```python
from build123d import *

# Parameters (mm, degrees)
BOSS_EXTRUDE1_DEPTH = 6
SKETCH2_R           = 1.125
SKETCH2_R_2         = 1.35
CUT_EXTRUDE1_DEPTH  = 7


with BuildPart() as part:
    # Sketch1 → Boss-Extrude1 (new body)
    with BuildSketch(Plane(origin=(0, 0, 0), x_dir=(1, 0, 0), z_dir=(0, 1, 0))):
        with BuildLine():
            Line((-12, 3.875), (12, 3.875))
            ThreePointArc((12, 3.875), (14.121320344, 2.996320344), (15, 0.875))
            Line((15, 0.875), (15, -0.875))
            ThreePointArc((15, -0.875), (14.121320344, -2.996320344), (12, -3.875))
            Line((12, -3.875), (-12, -3.875))
            ThreePointArc((-12, -3.875), (-14.121320344, -2.996320344), (-15, -0.875))
            Line((-15, -0.875), (-15, 0.875))
            ThreePointArc((-15, 0.875), (-14.121320344, 2.996320344), (-12, 3.875))
        make_face()
    extrude(amount=BOSS_EXTRUDE1_DEPTH)

    # Sketch2 → Cut-Extrude1 (cut, through all)
    with BuildSketch(Plane(origin=(0, 6, 0), x_dir=(1, 0, 0), z_dir=(0, 1, 0))):
        with Locations((-10, 0)):
            Circle(SKETCH2_R)
        with Locations((10, 0)):
            Circle(SKETCH2_R_2)
    extrude(amount=-CUT_EXTRUDE1_DEPTH, mode=Mode.SUBTRACT)


solid = part.part
```
The model under review builds one solid part; all positions refer to its coordinate system, in mm. Round coordinates to 2 decimals unless told otherwise and drop trailing zeros. Loops run counter-clockwise (first coordinate to the right, second up) from the corner with the lowest first, then second, coordinate; pieces in that order, holes last.
1) Consider section C-C on y = 1.1. State the section outline as (x, z) points (3 decimals), then the cut area to 3 significant figures.
Values follow:
outline: (-15, -0.875) arc R3 ccw to (-12, -3.875) - (12, -3.875) arc R3 ccw to (15, -0.875) - (15, 0.875) arc R3 ccw to (12, 3.875) - (-12, 3.875) arc R3 ccw to (-15, 0.875) - close; hole circle Ø2.25 at (-10, 0); hole circle Ø2.7 at (10, 0)
area: 215 mm2
2) Consider section B-B on z = 0. State the section outline as (x, y) points (3 decimals), then the cut area to 3 significant figures.
Values follow:
outline: (-15, 0) - (-11.125, 0) - (-11.125, 6) - (-15, 6) - close; (-8.875, 0) - (8.65, 0) - (8.65, 6) - (-8.875, 6) - close; (11.35, 0) - (15, 0) - (15, 6) - (11.35, 6) - close
area: 150 mm2
3) The part is to be moulded in two halves that separate along Z. For faces 1 (the face through (0, 0, 0)), 2 (the face through (-8.927, 3.042, -0.338)), 3 (the face through (0, 3, 3.875)), say which applies: pulls with the +Z half, pulls with the -Z half, needs draft (parallel to the pull), parting line crosses it, or undercut.
Values follow:
face 1: needs draft
face 2: undercut
face 3: pulls with the +Z half
4) Consider section D-D on z = 3. State the section outline as (x, y) points.
Values follow:
outline: (-14.12, 0) - (14.12, 0) - (14.12, 6) - (-14.12, 6) - close
5) Wall thickness on line 1 along X through (y, z) = (3.1, 0) (3 decimals); line 2 along Z through (x, y) = (-10, 2.25) (3 decimals); line 3 along X through (y, z) = (4.5, -0.5): over which ranges is each line inside the solid? List them lowest first.
Values follow:
line 1: x = -15 to -11.125, -8.875 to 8.65, 11.35 to 15
line 2: z = -3.875 to -1.125, 1.125 to 3.875
line 3: x = -15 to -11.01, -8.99 to 8.75, 11.25 to 15
6) Consider section A-A on x = -10. State the section outline as (y, z) points (3 decimals).
Values follow:
outline: (0, -3.875) - (6, -3.875) - (6, -1.125) - (0, -1.125) - close; (0, 1.125) - (6, 1.125) - (6, 3.875) - (0, 3.875) - close
7) Clearance check with a flat-ended pin moving along its axis: P1, Ø1, axis at y = 4.5, z = -2, coming from the +X side. State where the tip first meets the part, or that it passes through.
Values follow:
P1: stops at x = 14.93
